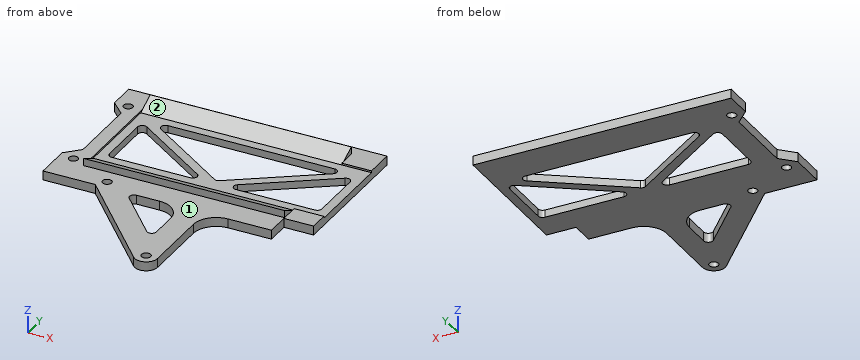
Autodesk Inventor part; units mm, degrees
ref_plane "YZ Plane" through (0, 0, 0) normal (1, 0, 0) x (0, 1, 0)
ref_plane "XZ Plane" through (0, 0, 0) normal (0, 1, 0) x (-1, 0, 0)
ref_plane "XY Plane" through (0, 0, 0) normal (0, 0, 1) x (1, 0, 0)
sketch "Sketch1" plane through (0, 0, 0) normal (0, 0, 1) x (1, 0, 0)
  line L0 (-26.0453, 15.4617) -> (23.9547, 15.4617)
  line L1 (23.9547, 15.4617) -> (23.9547, -18.5383)
  line L2 (23.9547, -18.5383) -> (-26.0453, -18.5383)
  line L3 (-26.0453, -18.5383) -> (-26.0453, 15.4617)
  point P0 (0, 0)
  dimension "d0" = 50
  dimension "d1" = 34
extrude "Extrusion1" add sketch "Sketch1" along normal blind 2
sketch "Sketch2" plane through (0, 0, 2) normal (0, 0, 1) x (1, 0, 0)
  line L0 (-26.0453, 15.4617) -> (-26.0453, -18.5383)
  line L1 (23.9547, 15.4617) -> (-26.0453, 15.4617)
  point P0 (0, 0)
  point P1 (-23.0453, 11.4617)
  point P2 (-23.0453, -11.5383)
  point P3 (-13.0453, -16.5383)
  dimension "d4" = 23
  dimension "d5" = 3
  dimension "d6" = 3
  dimension "d7" = 4
  dimension "d8" = 5
  dimension "d9" = 10
hole "Hole1" at (-23.0453, 11.4617, 2) at (-23.0453, -11.5383, 2) at (-13.0453, -16.5383, 2) direction (0, 0, -1) diameter 2 depth 6.5 tip angle 118
sketch "Sketch3" plane through (0, 0, 2) normal (0, 0, 1) x (1, 0, 0)
  line L0 (-26.0453, 15.4617) -> (-26.0453, -18.5383)
  line L1 (-26.0453, 8.4617) -> (-23.0453, 8.4617)
  line L2 (-23.0453, 8.4617) -> (-23.0453, -7.5383)
  line L3 (-23.0453, -7.5383) -> (-26.0453, -7.5383)
  line L4 (-26.0453, -7.5383) -> (-26.0453, 8.4617)
  line L5 (23.9547, 15.4617) -> (-26.0453, 15.4617)
  circle A0 centre (-23.0453, -11.5383) radius 1
  point P0 (0, 0)
  dimension "d17" = 7
  dimension "d18" = 4
  dimension "d19" = 3
extrude "Extrusion2" cut sketch "Sketch3" against normal blind 2 contours L1 L2 L3 L0
chamfer "Chamfer1" distance 3 angle 45 2 edges at (-26.0453, 8.4617, 1) (-26.0453, -7.5383, 1)
sketch "Sketch5" plane through (0, 0, 2) normal (0, 0, 1) x (1, 0, 0)
  line L0 (-20.0453, 14.9617) -> (23.9547, 14.9617)
  line L1 (23.9547, 14.9617) -> (23.9547, -13.0383)
  line L2 (23.9547, -13.0383) -> (-20.0453, -13.0383)
  line L3 (-20.0453, -13.0383) -> (-20.0453, 14.9617)
  line L4 (23.9547, 15.4617) -> (-26.0453, 15.4617)
  line L5 (-26.0453, -18.5383) -> (23.9547, -18.5383)
  line L6 (-23.0453, 8.4617) -> (-23.0453, -7.5383)
  line L7 (23.9547, -18.5383) -> (23.9547, 15.4617)
  circle A0 centre (-13.0453, -16.5383) radius 1
  point P0 (0, 0)
  dimension "d27" = 3
  dimension "d28" = 0
  dimension "d29" = 50
  dimension "d30" = 3.5
  dimension "d31" = 31.5
  dimension "d32" = 0.5
extrude "Extrusion3" cut sketch "Sketch5" against normal blind 0.4 contours L0 L1 L2 L3
sketch "Sketch8" plane through (0, 0, 2) normal (0, 0, 1) x (1, 0, 0)
  line L0 (-26.0453, -18.5383) -> (23.9547, -18.5383)
  line L1 (11.9547, -18.5383) -> (-1.0453, -18.5383)
  line L2 (-1.0453, -18.5383) -> (-1.0453, -44.5383)
  line L3 (-1.0453, -44.5383) -> (11.9547, -44.5383)
  line L4 (11.9547, -44.5383) -> (11.9547, -18.5383)
  line L5 (23.9547, -18.5383) -> (23.9547, 15.4617)
  circle A0 centre (-13.0453, -16.5383) radius 1
  line L6 (6.9547, -38.5383) -> (6.9547, -18.5383) construction
  line L7 (9.4547, -38.5383) -> (9.4547, -18.5383)
  line L8 (4.4547, -18.5383) -> (4.4547, -38.5383)
  arc A1 (4.4547, -38.5383) -> (9.4547, -38.5383) centre (6.9547, -38.5383) ccw
  arc A2 (9.4547, -18.5383) -> (4.4547, -18.5383) centre (6.9547, -18.5383) ccw
  circle A3 centre (6.9547, -38.5383) radius 1
  point P0 (0, 0)
  point P1 (23.9547, -13.0383)
  point P2 (6.9547, -28.5383)
  dimension "d48" = 12
  dimension "d49" = 25
  dimension "d50" = 20
  dimension "d51" = 22
  dimension "d52" = 6
  dimension "d53" = 5
  dimension "d54" = 2
extrude "Extrusion6" add sketch "Sketch8" against normal blind 2 contours L0 L7 A1 L8
fillet "Fillet1" radius 5 2 edges at (4.4547, -18.5383, 1) (9.4547, -18.5383, 1)
sketch "Sketch9" plane through (0, 0, 2) normal (0, 0, 1) x (1, 0, 0)
  circle A0 centre (-13.0453, -16.5383) radius 1
  circle A1 centre (6.9547, -38.5383) radius 1
  line L0 (-13.0453, -16.5383) -> (6.9547, -38.5383) construction
  line L1 (-14.8951, -18.22) -> (5.1049, -40.22)
  line L2 (8.8046, -36.8566) -> (-11.1954, -14.8566)
  arc A2 (-11.1954, -14.8566) -> (-14.8951, -18.22) centre (-13.0453, -16.5383) ccw
  arc A3 (5.1049, -40.22) -> (8.8046, -36.8566) centre (6.9547, -38.5383) ccw
  line L3 (-26.0453, -18.5383) -> (-0.5453, -18.5383)
  line L4 (-14.6058, -18.5383) -> (-7.8485, -18.5383)
  line L5 (4.4547, -23.5383) -> (4.4547, -38.5383)
  line L6 (4.4547, -32.0718) -> (4.4547, -38.5383)
  line L7 (4.4547, -38.5383) -> (6.7171, -41.027)
  arc A4 (4.4547, -38.5383) -> (9.4547, -38.5383) centre (6.9547, -38.5383) ccw
  point P0 (0, 0)
  point P1 (-3.0453, -27.5383)
extrude "Extrusion7" add sketch "Sketch9" against normal blind 2 contours L3 L2 L5 A4 L1
fillet "Fillet2" radius 1 2 edges at (-7.8485, -18.5383, 1) (4.4547, -32.0718, 1)
sketch "Sketch10" plane through (-26.0453, 15.4617, 0) normal (0, 1, 0) x (1, 0, 0)
  line L0 (50, 0) -> (50, -2)
  line L1 (0, 0) -> (0, -2)
  line L2 (50, -2) -> (0, -2)
  line L3 (0, -2) -> (0, 0)
  line L4 (0, 0) -> (50, 0)
  line L5 (50, 0) -> (50, -2)
  point P0 (26.0453, 0)
extrude "Extrusion8" add sketch "Sketch10" along normal blind 2
sketch "Sketch13" plane through (23.9547, -18.5383, 2) normal (1, 0, 0) x (0, 0, -1)
  line L0 (0, 0) -> (0, 5.5)
  line L1 (0.4, 5.5) -> (0.4, 33.5)
  line L2 (0.4, 5.5) -> (0, 5.5)
  line L3 (-1.6, 5.5) -> (0.4, 9.5)
  line L4 (0, 5.5) -> (0.4, 5.5)
  line L5 (-1.6, 5.5) -> (0.4, 5.5)
  line L6 (0.4, 5.5) -> (0.4, 9.5)
  point P0 (2, 18.5383)
  point P1 (0.4, 30.4)
  dimension "d70" = 1.6
  dimension "d71" = 4
extrude "Extrusion11" add sketch "Sketch13" against normal blind 44
sketch "Sketch14" plane through (23.9547, -18.5383, 2) normal (1, 0, 0) x (0, 0, -1)
  line L0 (0, 33.5) -> (0, 36)
  line L1 (0.4, 33.5) -> (0.4, 9.5)
  line L2 (0, 33.5) -> (0.4, 33.5)
  line L3 (-1.6, 33.5) -> (0.4, 29.5)
  line L4 (-1.6, 33.5) -> (0.4, 33.5)
  line L5 (0.4, 29.5) -> (0.4, 33.5)
  point P0 (2, 18.5383)
  dimension "d74" = 1.6
  dimension "d75" = 4
extrude "Extrusion12" add sketch "Sketch14" against normal blind 44
sketch "Sketch15" plane through (0, 0, 0) normal (0, 0, -1) x (-1, 0, 0)
  line L0 (-23.9547, -18.5383) -> (-23.9547, 17.4617)
  line L1 (-23.9547, 17.4617) -> (-30.4547, 17.4617)
  line L2 (-30.4547, 17.4617) -> (-30.4547, -13.3383)
  line L3 (-30.4547, -13.3383) -> (-23.9547, -13.3383)
  line L4 (-23.9547, -13.3383) -> (-23.9547, 17.4617)
  line L5 (-14.4547, -18.5383) -> (-23.9547, -18.5383)
  point P0 (0, 0)
  dimension "d78" = 5.2
  dimension "d79" = 6.5
extrude "Extrusion13" add sketch "Sketch15" against normal blind 2
sketch "Sketch16" plane through (0, 0, 2) normal (0, 0, 1) x (1, 0, 0)
  line L0 (30.4547, -13.3383) -> (30.4547, 17.4617)
  line L1 (-20.0453, -9.0383) -> (23.9547, -9.0383)
  line L2 (30.4547, 10.9617) -> (-20.0453, 10.9617)
  line L3 (-20.0453, 10.9617) -> (-20.0453, -9.0383)
  line L4 (-20.0453, -9.0383) -> (30.4547, -9.0383)
  line L5 (30.4547, -9.0383) -> (30.4547, 10.9617)
  line L6 (23.9547, 10.9617) -> (-20.0453, 10.9617)
  point P0 (0, 0)
  point P1 (30.4547, -9.0383)
extrude "Extrusion14" cut sketch "Sketch16" against normal blind 0.4
sketch "Sketch17" plane through (0, 0, 1.6) normal (0, 0, 1) x (1, 0, 0)
  line L0 (28.4547, -7.0383) -> (-18.0453, -7.0383)
  line L1 (-18.0453, -7.0383) -> (-18.0453, 8.9617)
  line L2 (-18.0453, 8.9617) -> (28.4547, 8.9617)
  line L3 (28.4547, 8.9617) -> (28.4547, -7.0383)
  line L4 (30.4547, -9.0383) -> (23.9547, -9.0383)
  line L5 (23.9547, 10.9617) -> (30.4547, 10.9617)
  line L6 (30.4547, 10.9617) -> (30.4547, -9.0383)
  line L7 (-20.0453, -9.8383) -> (-20.0453, 11.7617)
  point P0 (0, 0)
  dimension "d84" = 2
  dimension "d85" = 2
  dimension "d86" = 2
  dimension "d87" = 2
extrude "Extrusion15" cut sketch "Sketch17" against normal blind 2
sketch "Sketch18" plane through (0, 0, 1.6) normal (0, 0, 1) x (1, 0, 0)
  line L0 (-18.0453, -7.0383) -> (28.4547, -7.0383)
  line L1 (28.4547, 8.9617) -> (-18.0453, 8.9617)
  line L2 (5.2047, -7.0383) -> (28.4547, 8.9617) construction
  line L3 (5.7716, -7.8621) -> (29.0216, 8.1379)
  line L4 (27.8878, 9.7855) -> (4.6378, -6.2145)
  arc A0 (4.6378, -6.2145) -> (5.7716, -7.8621) centre (5.2047, -7.0383) ccw
  arc A1 (29.0216, 8.1379) -> (27.8878, 9.7855) centre (28.4547, 8.9617) ccw
  line L5 (5.2047, -7.0383) -> (-18.0453, 8.9617) construction
  line L6 (5.7716, -6.2145) -> (-17.4784, 9.7855)
  line L7 (-18.6122, 8.1379) -> (4.6378, -7.8621)
  arc A2 (4.6378, -7.8621) -> (5.7716, -6.2145) centre (5.2047, -7.0383) ccw
  arc A3 (-17.4784, 9.7855) -> (-18.6122, 8.1379) centre (-18.0453, 8.9617) ccw
  point P0 (0, 0)
  point P1 (16.5637, 8.9617)
  point P2 (-8.738, 9.9617)
  point P3 (16.8297, 0.9617)
  point P4 (-6.4203, 0.9617)
  point P5 (4.6378, -7.8621)
  point P6 (5.2047, -5.8244)
  dimension "d90" = 46.5
  dimension "d91" = 2
  dimension "d92" = 2
extrude "Extrusion16" add sketch "Sketch18" against normal blind 1.6 contours L7 A3 L6 L4 A0 L0 | L0 A0 L7 | A0 L4 L6 A2 L0 | L0 A2 A0 | A2 L6 L4 A1 L3 L0 | L0 L3 A2
fillet "Fillet3" radius 1 9 edges at (28.4547, -7.0383, 0.8) (28.4547, 7.7478, 0.8) (26.6907, 8.9617, 0.8) (6.9687, -7.0383, 0.8) (5.2047, -5.8244, 0.8) (3.4407, -7.0383, 0.8) (-16.2813, 8.9617, 0.8) (-18.0453, 7.7478, 0.8) (-18.0453, -7.0383, 0.8)
Input: part model. Units: mm. Frame: model coordinates. Face numbers are marked on the shaded views. Coordinates: 2 decimals unless noted, no trailing zeros. Order: outer loops, then holes, each group sorted by start corner. A loop starts at its lowest first (then second) coordinate and runs counter-clockwise, first axis right, second up. Notation, with made-up numbers: M -21,32 L 9,32 A21 cw 9,57 Z; hole C 50,-31.5 d2. An arc over 180 degrees is marked long. Write item = value, one per line. Start each with the question number.
(1) Section A-A on y = -4.5. Output: boundary loops of the cut face in (x, z).
(2) First-contact query: P1, Ø1.3, axis at y = 13.5, z = 3, coming from the -X side; P2, Ø1.3, axis at x = 0, z = 1, coming from the -Y side; P3, Ø16, axis at x = 1, y = 3.5, coming from the +Z side. Flat tips, straight axial feed; report the tip coordinate or a pass-through.
(3) Line query: line 1 along Y through (x, z) = (22, 0.3); line 2 along Y through (x, z) = (0, 1.35); line 3 along Y through (x, z) = (3.5, 0.9). Output: solid intervals per line, ascending. Write a range as [from, to].
(4) Section D-D on y = -27. Output: boundary loops of the cut face in (x, z), and give its area (3 significant figures).
(5) Section B-B on z = 3. Output: boundary loops of the cut face in (x, y).
(6) Pull-direction query (Y, two-part tool) for the marked faces 1 and 2; classes: released by +Y, released by -Y, zero draft, split by the parting line, or undercut.
(7) Section C-C on x = 13. Output: boundary loops of the cut face in (y, z), and give its area (3 significant figures).
Result set:
q1.outline = M -23.05,0 L -18.05,0 L -18.05,1.6 L -20.05,1.6 L -20.05,2 L -23.05,2 Z; M -0.25,0 L 3.28,0 L 3.28,1.6 L -0.25,1.6 Z; M 7.13,0 L 10.66,0 L 10.66,1.6 L 7.13,1.6 Z; M 28.45,0 L 30.45,0 L 30.45,1.6 L 28.45,1.6 Z
q2.P1 = -20.05
q2.P2 = -35.32
q2.P3 = 1.87
q3.line_1 = [-18.54, -7.04], [3.31, 5.73], [8.96, 17.46]
q3.line_2 = [-34.6, -27.17], [-18.57, -7.04], [-4.67, -2.24], [8.96, 17.46]
q3.line_3 = [-38.45, -30.48], [-20.6, -4.65], [8.96, 17.46]
q4.outline = M -6.91,0 L -0.16,0 L -0.16,2 L -6.91,2 Z; M 4.45,0 L 9.45,0 L 9.45,2 L 4.45,2 Z
q4.area = 23.5 mm²
q5.outline = M -20.05,-13.04 L 23.95,-13.04 L 23.95,-11.84 L -20.05,-11.84 Z; M -20.05,13.76 L 23.95,13.76 L 23.95,14.96 L -20.05,14.96 Z
q6.face_1 = zero draft
q6.face_2 = undercut
q7.outline = M -18.75,0 L -7.04,0 L -7.04,1.6 L -9.04,1.6 L -13.04,3.6 L -13.04,2 L -18.75,2 Z; M -2.89,0 L -0.46,0 L -0.46,1.6 L -2.89,1.6 Z; M 8.96,0 L 17.46,0 L 17.46,2 L 14.96,2 L 14.96,3.6 L 10.96,1.6 L 8.96,1.6 Z
q7.area = 47.5 mm²
